```python
from build123d import *

# Parameters (mm, degrees)
SKETCH_2_R          = 1.5
CUT_EXTRUDE_1_DEPTH = 10


with BuildPart() as part:
    # Эскиз1 → Повернуть1 (revolve)
    with BuildSketch(Plane.XY, mode=Mode.PRIVATE) as revolve_1_sk:
        Polygon((-17, 0), (-17, 25), (-16, 26), (-14, 26), (-14, 24), (-11, 24), (-9, 22), (-7, 24), (-5, 24), (-5, 22), (-2.5, 22), (-2.5, 24), (-0.5, 24), (0, 23.5), (0, 0), align=None)
    revolve(revolve_1_sk.sketch.rotate(Axis((0, 0, 0), (1, 0, 0)), 90), axis=Axis((0, 0, 0), (1, 0, 0)))

    # Эскиз2 → Вырез-Вытянуть1 (cut)
    with BuildSketch(Plane(origin=(0, 0, 0), x_dir=(0, 0, -1), z_dir=(1, 0, 0))):
        with Locations((0, 15.75)):
            Circle(SKETCH_2_R)
        with Locations((15.75, 0)):
            Circle(SKETCH_2_R)
        with Locations((-15.75, 0)):
            Circle(SKETCH_2_R)
        with Locations((0, -15.75)):
            Circle(SKETCH_2_R)
    extrude(amount=-CUT_EXTRUDE_1_DEPTH, mode=Mode.SUBTRACT)


solid = part.part
```
The listing builds one solid part. Answer for the finished solid, in the listing's coordinates (mm). A direction names the side the tool comes from. Coordinates: 2 decimals unless noted, no trailing zeros. Loops run counter-clockwise (first coordinate to the right, second up) from the corner with the lowest first, then second, coordinate; pieces in that order, holes last. Notation, with made-up numbers: M 46.5,-0.5 L 104.5,-0.5 A29 ccw 104.5,24.5 Z; hole C 47.5,69 d11. An arc over 180 degrees is marked long. Answer as CSV lines item,"result". Start each with the question number.
(1) Find the intervals of material crossed by L1, parallel to Y at x = -2.75, z = 0; L2, parallel to Y at x = -6.75, z = 0; L3, parallel to X at y = 18, z = -14, in increasing order. Write a range as [from, to].
(2) For faces 1 (the conical face through (-8.875, -6.646, 21.103)), 2 (the flat face through (-14, 23, 8)), 3 (the cylindrical face through (-14.986, 15.821, -20.633)), determine the directions among +Z, -Z, +X, -X, +Y, -Y from which every point of the face is accessible in a straight line to the end or side of a thin tool.
(3) The mould has two halves that part along Y. Classify faces 4 (the cylindrical face through (-5.99, -7.21, 22.89)), 5 (the cylindrical face through (-4.93, 16.76, 1.11)), 6 (the flat face through (-5, 21.2, 7)): pulls with the +Y half, pulls with the -Y half, needs draft (parallel to the pull), parting line crosses it, or undercut.
(4) The part is cut by section B-B (x = -1.75). Give the vertices of the cut face in (y, z), and give its area (3 significant figures).
(5) Given pin 1 (6 mm diameter, centred on x = -5, y = 5.5, fed in from +Z); pin 2 (8 mm diameter, centred on x = -8.5, z = 3.5, fed in from -Y); pin 3 (3 mm diameter, centred on x = -8.5, y = 14.5, fed in from -Z) (3 decimals), each flat-ended and moving along its own axis, determine where each tip first touches the part or whether it passes through.
Determined:
1,L1,"[-22, -17.25], [-14.25, 14.25], [17.25, 22]"
1,L2,"[-24, -17.25], [-14.25, 14.25], [17.25, 24]"
1,L3,"[-17, -9.8], [-8.2, -5], [-2.5, 0]"
2,face 1,"none"
2,face 2,"+X"
2,face 3,"+X, -X"
3,face 4,"parting line crosses it"
3,face 5,"undercut"
3,face 6,"needs draft"
4,outline,"C 0,0 d48; hole C -15.75,0 d3; hole C 0,-15.75 d3; hole C 0,15.75 d3; hole C 15.75,0 d3"
4,area,"1,780 mm2"
5,pin 1,"z = 23.87"
5,pin 2,"y = -24"
5,pin 3,"z = -19.425"
